Could you check a few things on this model? Use its own coordinates, in mm. A direction names the side the tool comes from. Round coordinates to 2 decimals unless told otherwise and drop trailing zeros. Loops run counter-clockwise (first coordinate to the right, second up) from the corner with the lowest first, then second, coordinate; pieces in that order, holes last.
from build123d import *

# Parameters (mm, degrees)
SKETCH_1_R            = 1
EXTRUDE_1_DEPTH       = 2
HOLE_WIZARD_M51_D     = 4.2
HOLE_WIZARD_M51_DEPTH = 14
HOLE_WIZARD_M51_TIP   = 1.2618073


with BuildPart() as part:
    # Эскиз1 → Бобышка-Вытянуть1 (new body)
    with BuildSketch(Plane(origin=(0, 0, 0), x_dir=(1, 0, 0), z_dir=(0, 1, 0))):
        with BuildLine():
            Line((0, 0), (20, 0))
            Line((20, 0), (20, 40.5))
            Line((20, 40.5), (19, 41.5))
            Line((19, 41.5), (14, 41.5))
            Line((14, 41.5), (14, 33.5))
            ThreePointArc((14, 33.5), (10, 29.5), (6, 33.5))
            Line((6, 33.5), (6, 41.5))
            Line((6, 41.5), (1, 41.5))
            Line((1, 41.5), (0, 40.5))
            Line((0, 40.5), (0, 0))
        make_face()
        with Locations(Location((10, 7, 0), (0, 0, 270))):
            Circle(SKETCH_1_R, mode=Mode.SUBTRACT)
    extrude(amount=EXTRUDE_1_DEPTH)

    # Отверстие обработанное метчиком M51
    with Locations(Plane(origin=(0, 2, 0), x_dir=(1, 0, 0), z_dir=(0, 1, 0))):
        with Locations((10, 7)):
            Hole(HOLE_WIZARD_M51_D / 2, depth=HOLE_WIZARD_M51_DEPTH)
            with Locations((0, 0, -(HOLE_WIZARD_M51_DEPTH + HOLE_WIZARD_M51_TIP / 2))):  # 118° drill point
                Cone(0, HOLE_WIZARD_M51_D / 2, HOLE_WIZARD_M51_TIP, mode=Mode.SUBTRACT)


solid = part.part
Item 1: If I drill on line 1 along Z through (x, y) = (10, 1.25); line 2 along Z through (x, y) = (7.5, 1); line 3 along X through (y, z) = (1.1, -33), over which ranges is the centre line in solid material (lowest first)?
Results list:
line 1: z = -29.5 to -9.1, -4.9 to 0
line 2: z = -30.38 to 0
line 3: x = 0 to 6.03, 13.97 to 20
Item 2: If we section it at B-B, the plane y = 1.5: Please give me the cut outline in (x, z), then the cut area to 3 significant figures.
Results list:
outline: (0, -40.5) - (1, -41.5) - (6, -41.5) - (6, -33.5) arc R4 cw to (14, -33.5) - (14, -41.5) - (19, -41.5) - (20, -40.5) - (20, 0) - (0, 0) - close; hole circle Ø4.2 at (10, -7)
area: 726 mm2
Item 3: If we section it at A-A, the plane z = -7: Please give me the cut outline in (x, y).
Results list:
outline: (0, 0) - (7.9, 0) - (7.9, 2) - (0, 2) - close; (12.1, 0) - (20, 0) - (20, 2) - (12.1, 2) - close
Item 4: We'd pull the mould along Z, two halves only. Please class faces 3 (the flat face through (10, 2, -21)), 4 (the cylindrical face through (11.548, 0.986, -8.419)), 5 (the cylindrical face through (10.1, 1, -29.5)): released by +Z, released by -Z, zero draft, split by the parting line, or undercut.
Results list:
face 3: zero draft
face 4: undercut
face 5: released by -Z
Item 5: If we section it at C-C, the plane z = -36.5: Please give me the cut outline in (x, y).
Results list:
outline: (0, 0) - (6, 0) - (6, 2) - (0, 2) - close; (14, 0) - (20, 0) - (20, 2) - (14, 2) - close
Item 6: For faces 1 (the flat face through (4, 1, -41.5)), 2 (the flat face through (6, 1, -37)), which set-ups out of +Z, -Z, +X, -X, +Y, -Y let a thin tool reach every point of the face, with its end or its side?
Results list:
face 1: -Z, +X, -X, +Y, -Y
face 2: -Z, +Y, -Y
